from build123d import *

# Parameters (mm, degrees)
SKETCH2_W           = 132
SKETCH2_H           = 82
SKETCH2_R           = 2.0066
SKETCH2_R_2         = 1.973275495
SKETCH2_R_3         = 2.037679125
SKETCH2_R_4         = 1.940146634
SKETCH2_R_5         = 7
SKETCH2_W_2         = 3
SKETCH2_H_2         = 40
SKETCH2_W_3         = 60
SKETCH2_H_3         = 3
BOSS_EXTRUDE1_DEPTH = 3


with BuildPart() as part:
    # Sketch2 → Boss-Extrude1 (new body)
    with BuildSketch(Plane(origin=(0, 0, 0), x_dir=(1, 0, 0), z_dir=(0, 1, 0))):
        with Locations((-60, 35)):
            Rectangle(SKETCH2_W, SKETCH2_H)
        with Locations(Location((-109.92679739, 63.113788195, 0), (0, 0, 270))):
            Circle(SKETCH2_R, mode=Mode.SUBTRACT)
        with Locations(Location((-110.18079739, 4.154783893, 0), (0, 0, 270))):
            Circle(SKETCH2_R_2, mode=Mode.SUBTRACT)
        with Locations(Location((-4.004277447, 63.080540095, 0), (0, 0, 270))):
            Circle(SKETCH2_R_3, mode=Mode.SUBTRACT)
        with Locations(Location((-4.720233043, 3.837756232, 0), (0, 0, 270))):
            Circle(SKETCH2_R_4, mode=Mode.SUBTRACT)
        with Locations(Location((-21.78879739, 49.11107203, 0), (0, 0, 270))):
            Circle(SKETCH2_R_5, mode=Mode.SUBTRACT)
        with Locations(Location((-21.78879739, 30.315787724, 0), (0, 0, 270))):
            Circle(SKETCH2_R_5, mode=Mode.SUBTRACT)
        with Locations(Location((-21.78879739, 12.028484075, 0), (0, 0, 270))):
            Circle(SKETCH2_R_5, mode=Mode.SUBTRACT)
        with Locations((1.5, 35)):
            Rectangle(SKETCH2_W_2, SKETCH2_H_2, mode=Mode.SUBTRACT)
        with Locations((-121.5, 35)):
            Rectangle(SKETCH2_W_2, SKETCH2_H_2, mode=Mode.SUBTRACT)
        with Locations((-60, 71.5)):
            Rectangle(SKETCH2_W_3, SKETCH2_H_3, mode=Mode.SUBTRACT)
        with Locations((-60, -1.5)):
            Rectangle(SKETCH2_W_3, SKETCH2_H_3, mode=Mode.SUBTRACT)
    extrude(amount=BOSS_EXTRUDE1_DEPTH)


solid = part.part
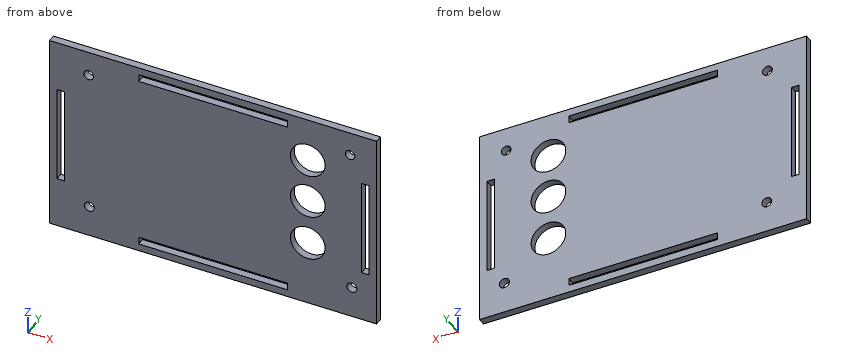
Design review of the part built by this model. Coordinates are the model's own, in mm. Give positions to 0.01 mm unless a question says otherwise; leave off trailing zeros. Write each loop counter-clockwise with the first axis right and the second up, starting at its lowest first coordinate (ties: lowest second). Pieces come first, ordered by that corner, then holes. Notation, with made-up numbers: M 14.5,-5.5 L 26.5,-5.5 A26 ccw 26.5,15.5 Z; hole C -11.5,-16 d5. An arc over 180 degrees is marked long. Return JSON: item names as keys, results as strings. Group by question number.
Item 1: Take a section at D-D (z = -8). Give the boundary of the cut face in (x, y).
Item 2: Take a section at A-A (x = -63.5). Give the boundary of the cut face in (y, z), plus the area to 3 significant figures.
Item 3: Take a section at B-B (z = -25). Give the boundary of the cut face in (x, y).
Item 4: Clearance check with a flat-ended pin moving along its axis: pin 1 Ø3 at (x, z) = (-110.18, -4.15) entering from -Y. State where the tip first meets the part, or that it passes through.
Item 5: Wall thickness on line 1 along X through (y, z) = (1.8, -21); line 2 along Z through (x, y) = (-62, 0.4); line 3 along X through (y, z) = (2.8, -71): over which ranges is each line inside the solid? List them lowest first.
Item 6: Take a section at C-C (y = 2.35). Count the separate pieces of the cut face and the enclosed holes in it, plus the area to 3 significant figures.
Return value:
{
 "1": {"outline": "M -126,0 L -27.51,0 L -27.51,3 L -126,3 Z; M -16.06,0 L 6,0 L 6,3 L -16.06,3 Z"},
 "2": {"outline": "M 0,-76 L 3,-76 L 3,-73 L 0,-73 Z; M 0,-70 L 3,-70 L 3,0 L 0,0 Z; M 0,3 L 3,3 L 3,6 L 0,6 Z", "area": "228 mm2"},
 "3": {"outline": "M -126,0 L -123,0 L -123,3 L -126,3 Z; M -120,0 L -26.34,0 L -26.34,3 L -120,3 Z; M -17.23,0 L 0,0 L 0,3 L -17.23,3 Z; M 3,0 L 6,0 L 6,3 L 3,3 Z"},
 "4": {"pin 1": "passes through"},
 "5": {"line 1": "x = -126 to -123, -120 to 0, 3 to 6", "line 2": "z = -76 to -73, -70 to 0, 3 to 6", "line 3": "x = -126 to -90, -30 to 6"},
 "6": {"separate pieces": "1", "enclosed holes": "11", "area": "9,710 mm2"}
}
